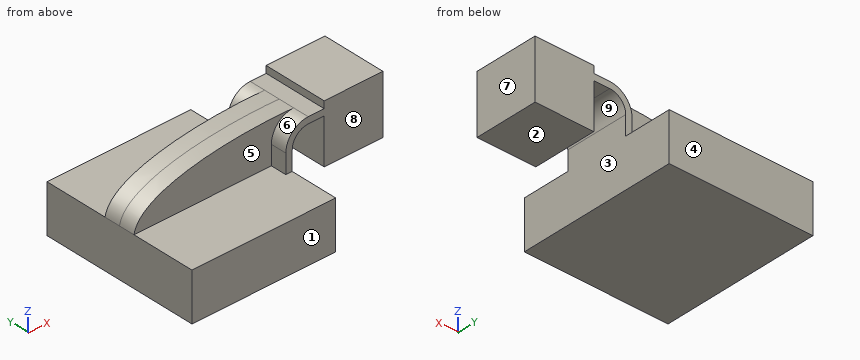
from build123d import *

# Parameters (mm, degrees)
F1_DEPTH = 63.5
F2_DEPTH = 12.7
F3_DEPTH = 25.4


with BuildPart() as f1:
    # F0 (on Front) → F1 (new body, symmetric)
    with BuildSketch(Plane.XZ):
        Polygon((57.15, -19.05), (57.15, 19.05), (52.07, 19.05), (-57.15, 19.05), (-57.15, -19.05), align=None)
    extrude(amount=F1_DEPTH, both=True)

    # F0 (on Front) → F2 (join, symmetric)
    with BuildSketch(Plane.XZ):
        with BuildLine():
            Line((-57.15, 19.05), (52.07, 19.05))
            Line((52.07, 19.05), (52.07, 34.29))
            ThreePointArc((52.07, 34.29), (57.277641, 46.862359), (69.85, 52.07))
            add(Edge.make_bspline(
                [(-57.15, 19.05), (-52.152008, 47.089871), (23.740247, 53.854882), (69.85, 52.07)],
                knots=[0, 0, 0, 0, 131.222408, 131.222408, 131.222408, 131.222408], degree=3))
        make_face()
    extrude(amount=F2_DEPTH, both=True)

    # F0 (on Front) → F3 (join, symmetric)
    with BuildSketch(Plane.XZ):
        Polygon((82.55, 52.07), (82.55, 46.99), (82.55, 10.928008), (129.273983, 10.928008), (129.273983, 57.651992), (82.55, 57.651992), align=None)
        with BuildLine():
            Line((52.07, 19.05), (57.15, 19.05))
            Line((57.15, 19.05), (57.15, 34.29))
            ThreePointArc((57.15, 34.29), (60.869744, 43.270256), (69.85, 46.99))
            Line((69.85, 46.99), (82.55, 46.99))
            Line((82.55, 46.99), (82.55, 52.07))
            Line((82.55, 52.07), (69.85, 52.07))
            ThreePointArc((69.85, 52.07), (57.277641, 46.862359), (52.07, 34.29))
            Line((52.07, 34.29), (52.07, 19.05))
        make_face()
    extrude(amount=F3_DEPTH, both=True)


solid = f1.part
Build history of the part. All positions in model axes, mm. Face numbers are marked on the shaded views. A direction names the side the tool comes from. Round coordinates to 2 decimals unless told otherwise and drop trailing zeros. Loops run counter-clockwise (first coordinate to the right, second up) from the corner with the lowest first, then second, coordinate; pieces in that order, holes last. Notation, with made-up numbers: (56, 33.25) -> (83, 33.25) arc R23 cw to (83, 71.25) -> close; hole circle Ø1 at (-26, 40.25). An arc over 180 degrees is marked (long way). One line per item, written item: value. Start each with the question number.
Q1. Cut at B-B on x = 101.5. List the corners of the cut face in (y, z), plus the area to 3 significant figures.
Q2. Probe line 1 along X through (y, z) = (18, 32); line 2 along X through (y, z) = (-3, 18.5); line 3 along Y through (x, z) = (-1.5, 35.5). List the from-to ranges inside material, lowest first.
Q3. 3-axis set-ups, long thin cutter, end or side, ignore diameter. For the marked faces 1, 2, 3, 4 and 5: which of +Z, -Z, +X, -X, +Y, -Y reach the whole face in a straight line?
Q4. Two-plate mould, pull along X, no slides. Class the marked faces 6, 7, 8 and 9: released by +X, released by -X, zero draft, split by the parting line, or undercut.
Q5. Cut at A-A on y = 23. List the corners of the cut face in (x, z), plus the area to 3 significant figures.
Q6. Drop flat-ended pins along their axis: pin 1 Ø16.5 at (x, z) = (31.5, 43.5) entering from +Y; pin 2 Ø15 at (x, y) = (5, 38) entering from +Z; pin 3 Ø6 at (y, z) = (-4, 56) entering from -X. Give the stop position or say it passes through.
Q7. Cut at C-C on z = 2. List the corners of the cut face in (x, y), plus the area to 3 significant figures.
Computed:
1. outline: (-25.4, 10.93) -> (25.4, 10.93) -> (25.4, 57.65) -> (-25.4, 57.65) -> close
1. area: 2,370 mm²
2. line 1: 52.07 to 57.15, 82.55 to 129.27
2. line 2: -57.15 to 57.15, 82.55 to 129.27
2. line 3: -12.7 to 12.7
3. face 1: +Z, -Z, +X, -X, -Y
3. face 2: -Z, +X, +Y, -Y
3. face 3: -Z, +Y, -Y
3. face 4: +Z, -Z, +X, -X, +Y
3. face 5: +Z, -X, -Y
4. face 6: released by -X
4. face 7: released by +X
4. face 8: zero draft
4. face 9: undercut
5. outline: (-57.15, -19.05) -> (57.15, -19.05) -> (57.15, 34.29) arc R12.7 cw to (69.85, 46.99) -> (82.55, 46.99) -> (82.55, 10.93) -> (129.27, 10.93) -> (129.27, 57.65) -> (82.55, 57.65) -> (82.55, 52.07) -> (69.85, 52.07) arc R17.78 ccw to (52.07, 34.29) -> (52.07, 19.05) -> (-57.15, 19.05) -> close
5. area: 6,800 mm²
6. pin 1: y = 12.7
6. pin 2: z = 19.05
6. pin 3: x = 82.55
7. outline: (-57.15, -63.5) -> (57.15, -63.5) -> (57.15, 63.5) -> (-57.15, 63.5) -> close
7. area: 14,500 mm²
